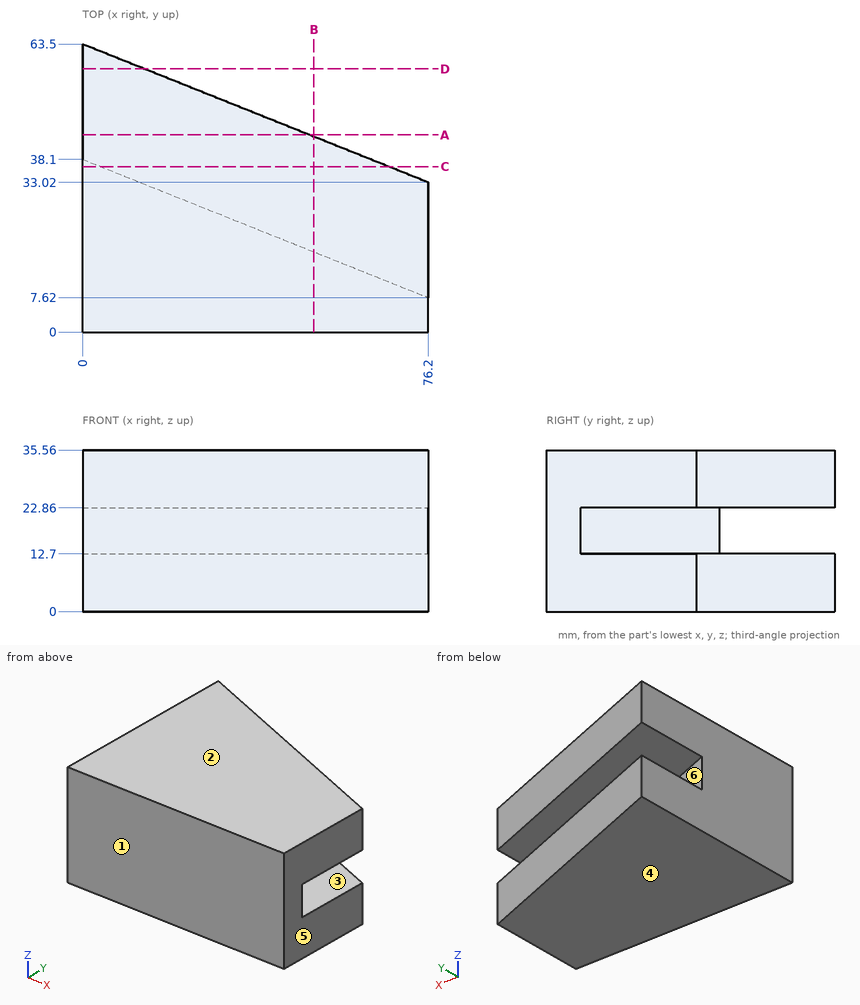
Could you check a few things on this drawing? It's one solid part, dimensions in mm from its lowest x, y, z. A direction names the side the tool comes from. Coordinates: 2 decimals unless noted, no trailing zeros. Loops run counter-clockwise (first coordinate to the right, second up) from the corner with the lowest first, then second, coordinate; pieces in that order, holes last. Notation, with made-up numbers: (9.25, -30.75) - (36.25, -30.75) arc R21 ccw to (36.25, 0.25) - close; hole circle Ø4 at (85.5, 38). An arc over 180 degrees is marked (long way). Return JSON: item names as keys, results as strings. Group by question number.
Item 1: If we section it at C-C on y = 36.5: Write out the boundary of the cut face in (x, z).
Item 2: Will these pins go through, and if not, where does the flat tip stop? P1, Ø8, axis at x = 61, y = 45, coming from the +Z side; P2, Ø1.5, axis at x = 48.5, z = 20, coming from the +Y side.
Item 3: If we section it at D-D on y = 58: Write out the boundary of the cut face in (x, z).
Item 4: We'd pull the mould along Z, two halves only. Please class the marked faces 1, 2, 3 and 4: +Z half, -Z half, draft (parallel to the pull), parting line (faces both ways), or undercut.
Item 5: On a 3-axis mill with a long thin cutter (end or side, diameter ignored), from which of +Z, -Z, +X, -X, +Y, -Y can I reach the whole of each face in a straight line? I mean the marked faces 5 and 6. Say none if no direction works.
Item 6: If we section it at B-B on x = 51: Write out the boundary of the cut face in (y, z).
Item 7: If we section it at A-A on y = 43.5: Write out the boundary of the cut face in (x, z).
Item 8: I need wall thicknesses on line 1 (Z direction, x = 47, y = 31); line 2 (Y direction, x = 40.5, z = 3); line 3 (Y direction, x = 52.5, z = 22). Which ranges of each line are inside material? Lowest first, please. Write a range as from..to.
Calculated:
{
 "1": {"outline": "(0, 0) - (67.5, 0) - (67.5, 12.7) - (4, 12.7) - (4, 22.86) - (67.5, 22.86) - (67.5, 35.56) - (0, 35.56) - close"},
 "2": {"P1": "passes through", "P2": "stops at y = 19"},
 "3": {"outline": "(0, 0) - (13.75, 0) - (13.75, 12.7) - (0, 12.7) - close; (0, 22.86) - (13.75, 22.86) - (13.75, 35.56) - (0, 35.56) - close"},
 "4": {"face 1": "draft", "face 2": "+Z half", "face 3": "undercut", "face 4": "-Z half"},
 "5": {"face 5": "+Z, -Z, +X, +Y, -Y", "face 6": "+X, +Y"},
 "6": {"outline": "(0, 0) - (43.1, 0) - (43.1, 12.7) - (17.7, 12.7) - (17.7, 22.86) - (43.1, 22.86) - (43.1, 35.56) - (0, 35.56) - close"},
 "7": {"outline": "(0, 0) - (50, 0) - (50, 12.7) - (0, 12.7) - close; (0, 22.86) - (50, 22.86) - (50, 35.56) - (0, 35.56) - close"},
 "8": {"line 1": "z = 0..12.7, 22.86..35.56", "line 2": "y = 0..47.3", "line 3": "y = 0..17.1"}
}
